Can you work these out from the model? Positions are in its coordinate system, mm. A direction names the side the tool comes from. Round coordinates to 2 decimals unless told otherwise and drop trailing zeros. Loops run counter-clockwise (first coordinate to the right, second up) from the corner with the lowest first, then second, coordinate; pieces in that order, holes last. Notation, with made-up numbers: (38, 7.5) -> (61, 7.5) arc R24 cw to (61, 45.5) -> close; hole circle Ø9 at (72.5, 44.25). An arc over 180 degrees is marked (long way). Write item = value, one per line.
from build123d import *

# Parameters (mm, degrees)
F1_DEPTH = 3
F2_D     = 4.1


with BuildPart() as f1:
    # F0 (on Top) → F1 (new body)
    with BuildSketch(Plane.XY):
        with BuildLine():
            Line((13.0338203524, 11), (-61.9661796476, 11))
            ThreePointArc((-61.9661796476, 11), (-72.9661796476, 0), (-61.9661796476, -11))
            Line((-61.9661796476, -11), (13.0338203524, -11))
            ThreePointArc((13.0338203524, -11), (22.4049554576, 0), (13.0338203524, 11))
        make_face()
        with BuildLine():
            ThreePointArc((-48.3821049507, -1.6), (-49.9821049507, 0), (-48.3821049507, 1.6))
            Line((-48.3821049507, 1.6), (17.6169872284, 1.6))
            ThreePointArc((17.6169872284, 1.6), (19.2169872284, 0), (17.6169872284, -1.6))
            Line((17.6169872284, -1.6), (-48.3821049507, -1.6))
        make_face(mode=Mode.SUBTRACT)
    extrude(amount=F1_DEPTH)

    # F2 (through all)
    with Locations(Plane(origin=(0, 0, 0), x_dir=(1, 0, 0), z_dir=(0, 0, -1))):
        with Locations((-65.4418841004, 0)):
            Hole(F2_D / 2)


solid = f1.part
1. Suppose I cut it at B-B, the plane x = -5.5. List the corners of the cut face in (y, z) for me, and give its area (3 significant figures).
Entries:
outline = (-11, 0) -> (-1.6, 0) -> (-1.6, 3) -> (-11, 3) -> close; (1.6, 0) -> (11, 0) -> (11, 3) -> (1.6, 3) -> close
area = 56.4 mm²
2. We'd pull the mould along Y, two halves only. Please class faces 1 (the cylindrical face through (-63.394, -0.09, 1.521)), 2 (the flat face through (-26, -2, 0)), 3 (the flat face through (-24, 11, 1)): released by +Y, released by -Y, zero draft, split by the parting line, or undercut.
Entries:
face_1 = undercut
face_2 = zero draft
face_3 = released by +Y
3. Suppose I cut it at D-D, the plane x = 14. List the corners of the cut face in (y, z) for me.
Entries:
outline = (-10.8, 0) -> (-1.6, 0) -> (-1.6, 3) -> (-10.8, 3) -> close; (1.6, 0) -> (10.8, 0) -> (10.8, 3) -> (1.6, 3) -> close
4. I'm going to push a flat-ended pin straight in: pin 1 (6 mm diameter, centred on x = -62.5, y = 2.5, fed in from -Z). Where does the tip first touch, or does it pass through?
Entries:
pin_1 = 0
5. Suppose I cut it at C-C, the plane z = 2.15. List the corners of the cut face in (x, y) for me.
Entries:
outline = (-61.97, -11) -> (13.03, -11) arc R11.14 ccw to (13.03, 11) -> (-61.97, 11) arc R11 ccw to start; hole circle Ø4.1 at (-65.44, 0); hole (-48.38, -1.6) -> (17.62, -1.6) arc R1.6 ccw to (17.62, 1.6) -> (-48.38, 1.6) arc R1.6 ccw to start
6. I need wall thicknesses on line 1 (Y direction, x = -10.5, z = 0.85); line 2 (X direction, y = -1, z = 2.7); line 3 (Y direction, x = 14, z = 1.35). Which ranges of each line are inside material? Lowest first, please. Write a range as [from, to].
Entries:
line_1 = [-11, -1.6], [1.6, 11]
line_2 = [-72.92, -67.23], [-63.65, -49.63], [18.87, 22.36]
line_3 = [-10.8, -1.6], [1.6, 10.8]
7. For faces 4 (the cylindrical face through (-72.964, 0.242, 1.479)), 5 (the flat face through (-16, 1.6, 1)), which set-ups out of +Z, -Z, +X, -X, +Y, -Y let a thin tool reach every point of the face, with its end or its side?
Entries:
face_4 = +Z, -Z, -X
face_5 = +Z, -Z
8. Suppose I cut it at A-A, the plane y = 0. List the corners of the cut face in (x, z) for me, and give its area (3 significant figures).
Entries:
outline = (-72.97, 0) -> (-67.49, 0) -> (-67.49, 3) -> (-72.97, 3) -> close; (-63.39, 0) -> (-49.98, 0) -> (-49.98, 3) -> (-63.39, 3) -> close; (19.22, 0) -> (22.4, 0) -> (22.4, 3) -> (19.22, 3) -> close
area = 66.2 mm²
